CAD build for the part. Positions are in the model's coordinates, mm. Face numbers are marked on the shaded views. A direction names the side the tool comes from. Give positions to 0.01 mm unless a question says otherwise; leave off trailing zeros. Loops run counter-clockwise (first coordinate to the right, second up) from the corner with the lowest first, then second, coordinate; pieces in that order, holes last. Notation, with made-up numbers: M 34,86.5 L 43,86.5 A26 ccw 43,120.5 Z; hole C 57.5,1 d3. An arc over 180 degrees is marked long. One line per question, with ' | ' between items.
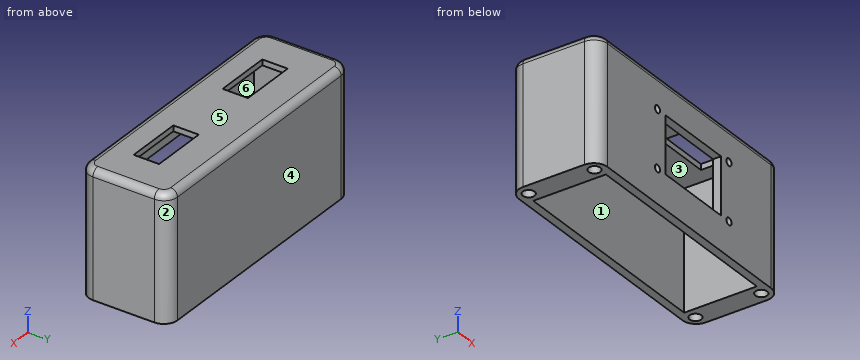
Autodesk Fusion 360 part; units mm, degrees
sketch "Sketch1" plane through (0, 0, 0) normal (0, 0, 1) x (1, 0, 0)
  line L0 (0, 0) -> (-115, 0)
  line L1 (-115, 0) -> (-115, 39)
  line L2 (-115, 39) -> (0, 39)
  line L3 (0, 39) -> (0, 0)
  circle A0 centre (-5, 34) radius 2.6
  circle A1 centre (-5, 34) radius 1.6
  circle A2 centre (-5, 5) radius 2.6
  circle A3 centre (-5, 5) radius 1.6
  circle A4 centre (-110, 5) radius 2.6
  circle A5 centre (-110, 5) radius 1.6
  circle A6 centre (-110, 34) radius 2.6
  circle A7 centre (-110, 34) radius 1.6
  line L4 (-10, 35.5) -> (-105, 35.5)
  line L5 (-105, 35.5) -> (-105, 3.5)
  line L6 (-105, 3.5) -> (-10, 3.5)
  line L7 (-10, 3.5) -> (-10, 35.5)
  dimension "d1" = 115
  dimension "d2" = 39
  dimension "d3" = 5.2
  dimension "d4" = 5
  dimension "d5" = 5
  dimension "d6" = 3.2
  dimension "d7" = 5.2
  dimension "d8" = 5
  dimension "d9" = 5
  dimension "d10" = 3.2
  dimension "d11" = 5.2
  dimension "d12" = 5
  dimension "d13" = 5
  dimension "d14" = 3.2
  dimension "d15" = 5.2
  dimension "d16" = 5
  dimension "d17" = 5
  dimension "d18" = 3.2
  dimension "d19" = 95
  dimension "d20" = 32
  dimension "d21" = 10
  dimension "d22" = 3.5
extrude "Extrude1" add sketch "Sketch1" along normal blind 55 contours L0 L1 L2 L3 | A0 | A1 | A2 | A3 | A4 | A5 | A6 | A7 | L4 L5 L6 L7
extrude "Extrude2" cut sketch "Sketch1" along normal blind 52.5 contours L4 L5 L6 L7
extrude "Extrude3" cut sketch "Sketch1" along normal blind 5 contours A0 | A2 | A4 | A6
extrude "Extrude4" cut sketch "Sketch1" along normal blind 15 contours A1 | A3 | A5 | A7
sketch "Sketch2" plane through (0, 0, 0) normal (0, 1, 0) x (1, 0, 0)
  line L0 (-27.5, -10) -> (-82.5, -10)
  line L1 (-82.5, -10) -> (-82.5, -45)
  line L2 (-82.5, -45) -> (-27.5, -45)
  line L3 (-27.5, -45) -> (-27.5, -10)
  line L4 (-37.5, -15) -> (-72.5, -15)
  line L5 (-72.5, -15) -> (-72.5, -40)
  line L6 (-72.5, -40) -> (-37.5, -40)
  line L7 (-37.5, -40) -> (-37.5, -15)
  circle A0 centre (-32.5, -15) radius 1.6
  circle A1 centre (-32.5, -40) radius 1.6
  circle A2 centre (-77.5, -15) radius 1.6
  circle A3 centre (-77.5, -40) radius 1.6
  line L8 (0, 0) -> (-115, 0)
  line L9 (0, 0) -> (0, -55)
  dimension "d31" = 55
  dimension "d32" = 35
  dimension "d33" = 35
  dimension "d34" = 25
  dimension "d35" = 10
  dimension "d36" = 5
  dimension "d37" = 3.2
  dimension "d38" = 5
  dimension "d39" = 5
  dimension "d40" = 3.2
  dimension "d41" = 5
  dimension "d42" = 5
  dimension "d43" = 3.2
  dimension "d44" = 5
  dimension "d45" = 5
  dimension "d46" = 3.2
  dimension "d47" = 5
  dimension "d48" = 5
  dimension "d49" = 10
  dimension "d50" = 27.5
extrude "Extrude5" cut sketch "Sketch2" along normal blind 15 contours L4 L5 L6 L7
extrude "Extrude6" cut sketch "Sketch2" along normal blind 10 contours A0 | A1 | A2 | A3
ref_plane "WorkPlane1" through (0, 0, 60) normal (0, 0, 1) x (1, 0, 0)
sketch "Sketch3" plane through (0, 0, 60) normal (0, 0, 1) x (1, 0, 0)
  line L0 (-98, 23.2) -> (-73, 23.2)
  line L1 (-73, 23.2) -> (-73, 12)
  line L2 (-73, 12) -> (-98, 12)
  line L3 (-98, 12) -> (-98, 23.2)
  line L4 (-42, 23.2) -> (-17, 23.2)
  line L5 (-17, 23.2) -> (-17, 12)
  line L6 (-17, 12) -> (-42, 12)
  line L7 (-42, 12) -> (-42, 23.2)
  line L8 (0, 39) -> (-115, 39)
  line L9 (-99, 30.7) -> (-72, 30.7)
  line L10 (-72, 30.7) -> (-72, 3.7)
  line L11 (-72, 3.7) -> (-99, 3.7)
  line L12 (-99, 3.7) -> (-99, 30.7)
  line L13 (-43, 30.7) -> (-16, 30.7)
  line L14 (-16, 30.7) -> (-16, 3.7)
  line L15 (-16, 3.7) -> (-43, 3.7)
  line L16 (-43, 3.7) -> (-43, 30.7)
  line L17 (-115, 0) -> (0, 0)
  line L18 (-115, 39) -> (-115, 0)
  line L19 (0, 0) -> (0, 39)
  dimension "d56" = 25
  dimension "d57" = 11.2
  dimension "d58" = 25
  dimension "d59" = 11.2
  dimension "d61" = 27
  dimension "d62" = 27
  dimension "d63" = 7.5
  dimension "d64" = 1
  dimension "d65" = 27
  dimension "d66" = 27
  dimension "d67" = 1
  dimension "d68" = 7.5
  dimension "d69" = 3.7
  dimension "d70" = 3.7
  dimension "d73" = 16
  dimension "d74" = 16
extrude "Extrude7" cut sketch "Sketch3" against normal blind 25 contours L0 L1 L2 L3 | L4 L5 L6 L7
fillet "Fillet1" radius 6 4 edges at (0, 39, 27.5) (-115, 39, 27.5) (0, 0, 27.5) (-115, 0, 27.5)
fillet "Fillet2" radius 3 8 edges at (-113.2426, 37.2426, 55) (-115, 19.5, 55) (-113.2426, 1.7574, 55) (-57.5, 0, 55) (-1.7574, 1.7574, 55) (0, 19.5, 55) (-1.7574, 37.2426, 55) (-57.5, 39, 55)
Item 1: Drill centre lines: line 1 along Y through (x, z) = (-81, 41.5); line 2 along Y through (x, z) = (-110, 2); line 3 along X through (y, z) = (14, 7). Where is each one in solid material? Low to high. Write a range as [from, to].
Conclusion:
line 1: [0, 3.5], [35.5, 39] | line 2: [0.08, 2.4], [7.6, 31.4], [36.6, 38.92] | line 3: [-115, -105], [-10, 0]
Item 2: 3-axis set-ups, long thin cutter, end or side, ignore diameter. For the marked faces 1 and 2: which of +Z, -Z, +X, -X, +Y, -Y reach the whole face in a straight line?
Conclusion:
face 1: -Z | face 2: +Z, -Z, +X, +Y
Item 3: Saw through at A-A on x = -32.5. Give the cut face in (y, z).
Conclusion:
outline: M 0,0 L 3.5,0 L 3.5,13.4 L 0,13.4 Z; M 0,16.6 L 3.5,16.6 L 3.5,38.4 L 0,38.4 Z; M 0,41.6 L 3.5,41.6 L 3.5,52.5 L 12,52.5 L 12,55 L 3,55 A3 ccw 0,52 Z; M 23.2,52.5 L 35.5,52.5 L 35.5,0 L 39,0 L 39,52 A3 ccw 36,55 L 23.2,55 Z
Item 4: Saw through at B-B on z = 44.5. Give the cut face in (x, y), and give its area (3 significant figures).
Conclusion:
outline: M -115,6 A6 ccw -109,0 L -6,0 A6 ccw 0,6 L 0,33 A6 ccw -6,39 L -109,39 A6 ccw -115,33 Z; hole M -105,3.5 L -10,3.5 L -10,35.5 L -105,35.5 Z | area: 1,410 mm²
Item 5: Saw through at D-D on y = 26. Give the cut face in (x, z).
Conclusion:
outline: M -115,0 L -105,0 L -105,52.5 L -10,52.5 L -10,0 L 0,0 L 0,52 A3 ccw -3,55 L -112,55 A3 ccw -115,52 Z
Item 6: Mould opens along Y. For the marked faces 3, 4, 5 and 6 say: pulls with the +Y half, pulls with the -Y half, needs draft (parallel to the pull), parting line crosses it, or undercut.
Conclusion:
face 3: undercut | face 4: pulls with the +Y half | face 5: needs draft | face 6: undercut
Item 7: Drop flat-ended pins along their axis: P1, Ø4, axis at x = -110, y = 33.5, coming from the -Z side; P2, Ø10, axis at x = -42.5, y = 10, coming from the -Z side; P3, Ø1.6, axis at x = -109.5, y = 5.5, coming from the -Z side. Give the stop position or say it passes through.
Conclusion:
P1: z = 5 | P2: z = 52.5 | P3: z = 15
Item 8: Saw through at C-C on x = -100. Give the cut face in (y, z).
Conclusion:
outline: M 0,0 L 3.5,0 L 3.5,52.5 L 35.5,52.5 L 35.5,0 L 39,0 L 39,52 A3 ccw 36,55 L 3,55 A3 ccw 0,52 Z
